```python
from build123d import *

# Parameters (mm, degrees)
ESQUISSE1_R        = 23.5
BOSS_EXTRU_1_DEPTH = 10


with BuildPart() as part:
    # Esquisse1 → Boss.-Extru.1 (new body)
    with BuildSketch(Plane.XY):
        with BuildLine():
            Line((0, 0), (190, 0))
            Line((190, 0), (198.660254038, 0))
            Line((198.660254038, 0), (190, 5))
            Line((190, 5), (80.841978046, 68.02241336))
            ThreePointArc((80.841978046, 68.02241336), (51.627444809, 71.868579626), (28.25, 53.930435314))
            Line((28.25, 53.930435314), (0, 5))
            Line((0, 5), (0, 0))
        make_face()
        with Locations((61.591978046, 34.680435314)):
            Circle(ESQUISSE1_R, mode=Mode.SUBTRACT)
    extrude(amount=BOSS_EXTRU_1_DEPTH)


solid = part.part
```
Input: part model. Units: mm. Frame: model coordinates. Coordinates: 2 decimals unless noted, no trailing zeros. Loops run counter-clockwise (first coordinate to the right, second up) from the corner with the lowest first, then second, coordinate; pieces in that order, holes last. Notation, with made-up numbers: (30.25, -30.75) - (76.25, -30.75) arc R35 cw to (76.25, 1.25) - close; hole circle Ø6 at (41, -35). An arc over 180 degrees is marked (long way). Answer in a Markdown table with one row per item.
(1) Cut plane A-A on y = 13. Output: boundary loops of the cut face in (x, z).
Model answer:
| item | result |
|---|---|
| outline | (4.62, 0) - (52.53, 0) - (52.53, 10) - (4.62, 10) - close; (70.66, 0) - (176.14, 0) - (176.14, 10) - (70.66, 10) - close |
(2) Cut plane B-B on z = 6.5. Output: boundary loops of the cut face in (x, y), plus the area to 3 significant figures.
Model answer:
| item | result |
|---|---|
| outline | (0, 0) - (198.66, 0) - (80.84, 68.02) arc R38.5 ccw to (28.25, 53.93) - (0, 5) - close; hole circle Ø47 at (61.59, 34.68) |
| area | 6,730 mm² |
(3) Pin query (flat end, axial travel): P1, Ø1.5, axis at y = 57.5, z = 3, coming from the +X side; P2, Ø3, axis at y = 62.5, z = 3, coming from the +X side. Return the tip coordinate at first contact, or that it passes through.
Model answer:
| item | result |
|---|---|
| P1 | stops at x = 100.37 |
| P2 | stops at x = 93.01 |
(4) Cut plane C-C on y = 49. Output: boundary loops of the cut face in (x, z).
Model answer:
| item | result |
|---|---|
| outline | (25.4, 0) - (42.96, 0) - (42.96, 10) - (25.4, 10) - close; (80.23, 0) - (113.79, 0) - (113.79, 10) - (80.23, 10) - close |
(5) Cut plane D-D on x = 173. Output: boundary loops of the cut face in (y, z), plus the area to 3 significant figures.
Model answer:
| item | result |
|---|---|
| outline | (0, 0) - (14.81, 0) - (14.81, 10) - (0, 10) - close |
| area | 148 mm² |
(6) Mould query, pull axis Y, two halves, no side actions, for faces 1 (the face through (14.323, 29.808, 4.93)), 2 (the face through (98, 0, 5)), 3 (the face through (56.5, 11.74, 4.93)). Classes: pulls with the +Y half, pulls with the -Y half, needs draft (parallel to the pull), parting line crosses it, or undercut.
Model answer:
| item | result |
|---|---|
| face 1 | pulls with the +Y half |
| face 2 | pulls with the -Y half |
| face 3 | undercut |
(7) Material intervals for L1, parallel to X at y = 38.5, z = 7.25; L2, parallel to X at y = 34.5, z = 9.5; L3, parallel to Y at x = 64, z = 5.5, sorted ascending. Write a range as from..to.
Model answer:
| item | result |
|---|---|
| L1 | x = 19.34..38.4, 84.78..131.98 |
| L2 | x = 17.03..38.09, 85.09..138.9 |
| L3 | y = 0..11.3, 58.06..73.11 |
